Study the drawing (mm; zero at the part's minimum x, y, z) and answer. A direction names the side the tool comes from. Round coordinates to 2 decimals unless told otherwise and drop trailing zeros. Loops run counter-clockwise (first coordinate to the right, second up) from the corner with the lowest first, then second, coordinate; pieces in that order, holes last. Notation, with made-up numbers: M 19.25,-14.75 L 72.25,-14.75 A11 cw 72.25,1.25 Z; hole C 77.25,64.5 d5. An arc over 180 degrees is marked long. Write each question's results on one line, items separated by ' | '.
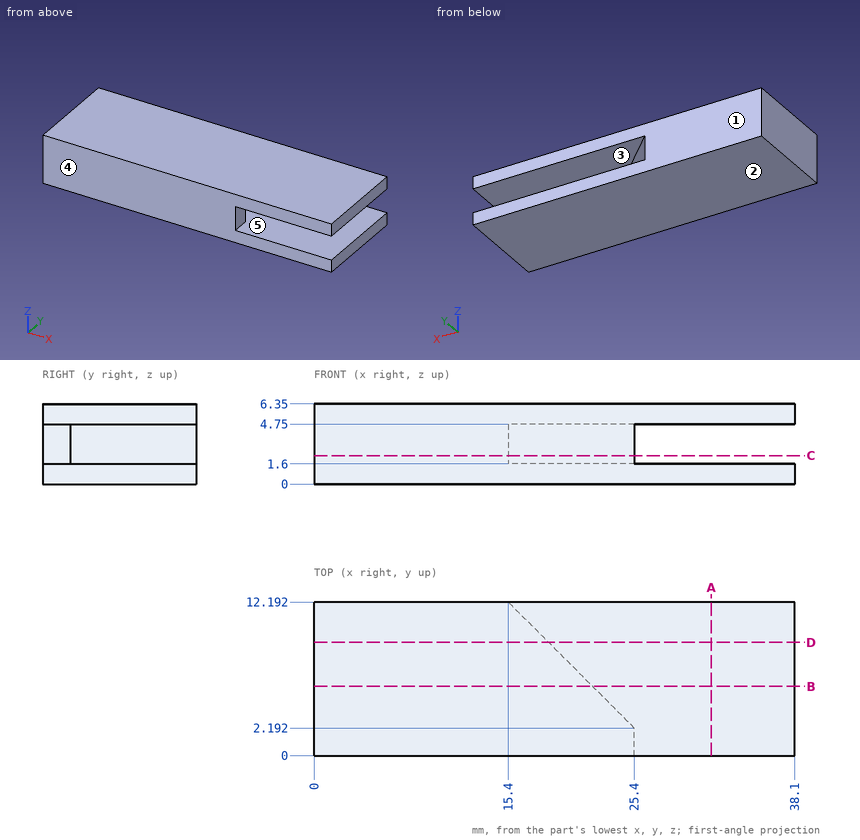
Item 1: The part is cut by section C-C (z = 2.25). Determine the outline of the cut face in (x, y).
Outcome:
outline: M 0,0 L 25.4,0 L 25.4,2.19 L 15.4,12.19 L 0,12.19 Z
Item 2: Flat-ended cylindrical pins translate along their axes: pin 1 (1 mm diameter, centred on y = 2, z = 3.5, fed in from -X); pin 2 (1.1 mm diameter, centred on y = 0.5, z = 2.5, fed in from +X). Find the tip coordinate at first contact, or state that the pin passes through.
Outcome:
pin 1: stops at x = 0 | pin 2: stops at x = 25.4
Item 3: The part is cut by section B-B (y = 5.5). Determine the outline of the cut face in (x, z).
Outcome:
outline: M 0,0 L 38.1,0 L 38.1,1.6 L 22.09,1.6 L 22.09,4.75 L 38.1,4.75 L 38.1,6.35 L 0,6.35 Z
Item 4: The mould has two halves that part along Z. Classify the marked faces 1, 2 and 3: pulls with the +Z half, pulls with the -Z half, needs draft (parallel to the pull), parting line crosses it, or undercut.
Outcome:
face 1: needs draft | face 2: pulls with the -Z half | face 3: undercut
Item 5: For the marked faces 4 and 5, determine the directions among +Z, -Z, +X, -X, +Y, -Y from which every point of the face is accessible in a straight line to the end or side of a thin tool.
Outcome:
face 4: +Z, -Z, +X, -X, -Y | face 5: +X, +Y
Item 6: The part is cut by section D-D (y = 9). Determine the outline of the cut face in (x, z).
Outcome:
outline: M 0,0 L 38.1,0 L 38.1,1.6 L 18.59,1.6 L 18.59,4.75 L 38.1,4.75 L 38.1,6.35 L 0,6.35 Z
Item 7: The part is cut by section A-A (x = 31.5). Determine the outline of the cut face in (y, z), plus the area to 3 significant figures.
Outcome:
outline: M 0,0 L 12.19,0 L 12.19,1.6 L 0,1.6 Z; M 0,4.75 L 12.19,4.75 L 12.19,6.35 L 0,6.35 Z | area: 39.0 mm2
Item 8: Straight lines are drawn through the part: line 1 (Z direction, x = 32, y = 1.25); line 2 (X direction, y = 1, z = 3.75); line 3 (Y direction, x = 19, z = 2.25). For each, find the intervals that lie inside material, in ascending order.
Outcome:
line 1: z = 0 to 1.6, 4.75 to 6.35 | line 2: x = 0 to 25.4 | line 3: y = 0 to 8.59
